The listing builds one solid part. Answer for the finished solid, in the listing's coordinates (mm). A direction names the side the tool comes from. Round coordinates to 2 decimals unless told otherwise and drop trailing zeros. Write each loop counter-clockwise with the first axis right and the second up, starting at its lowest first coordinate (ties: lowest second). Pieces come first, ordered by that corner, then holes. Notation, with made-up numbers: (3.25, -31) -> (37.25, -31) arc R26 ccw to (37.25, -12) -> close; hole circle Ø2 at (75, -20). An arc over 180 degrees is marked (long way). Write each question's results on one line, items separated by ' | '. Start each with the question number.
```python
from build123d import *

# Parameters (mm, degrees)
F1_DEPTH = 6
F2_R     = 6.5
F3_DEPTH = 6
F4_R     = 6.5
F5_DEPTH = 6


with BuildPart() as f1:
    # F0 (on Front) → F1 (new body)
    with BuildSketch(Plane.XZ):
        with BuildLine():
            Line((32, -12.5), (32, 12.5))
            Line((32, 12.5), (-32, 12.5))
            Line((-32, 12.5), (-32, 6.5))
            Line((-32, 6.5), (-12, 6.5))
            ThreePointArc((-12, 6.5), (-7.403806, 4.596194), (-5.5, 0))
            ThreePointArc((-5.5, 0), (-7.403806, -4.596194), (-12, -6.5))
            Line((-12, -6.5), (-32, -6.5))
            Line((-32, -6.5), (-32, -12.5))
            Line((-32, -12.5), (-12.5, -12.5))
            Line((-12.5, -12.5), (12.5, -12.5))
            Line((12.5, -12.5), (32, -12.5))
        make_face()
    extrude(amount=F1_DEPTH)

    # F2 (on face) → F3 (join)
    with BuildSketch(Plane.YZ.offset(32)):
        with BuildLine():
            Line((0, 12.5), (0, -12.5))
            Line((0, -12.5), (12, -12.5))
            ThreePointArc((12, -12.5), (24.5, 0), (12, 12.5))
            Line((12, 12.5), (0, 12.5))
        make_face()
        with Locations((12, 0)):
            Circle(F2_R, mode=Mode.SUBTRACT)
    extrude(amount=-F3_DEPTH)

    # F4 (on face) → F5 (join)
    with BuildSketch(Plane.XY.offset(12.5)):
        with BuildLine():
            Line((32, -18), (32, -6))
            Line((32, -6), (7, -6))
            Line((7, -6), (7, -18))
            ThreePointArc((7, -18), (19.5, -30.5), (32, -18))
        make_face()
        with Locations((19.5, -18)):
            Circle(F4_R, mode=Mode.SUBTRACT)
    extrude(amount=-F5_DEPTH)


solid = f1.part
```
Q1. Each of these flat-tipped pins is pushed along its axis until it touches: pin 1 (12.5 mm diameter, centred on x = 11, z = -6, fed in from +Y); pin 2 (8 mm diameter, centred on x = 12, y = -21, fed in from -Z); pin 3 (3 mm diameter, centred on x = -17, z = -6.5, fed in from -Y). Where does it stop, or does it pass through?
Q2. For faces 1 (the flat face through (-32, -3, -9)), 2 (the flat face through (25, -13, 6.5)), 3 (the flat face through (-22, -3, -6.5)), 4 (the flat face through (7, -12, 10)), 5 (the flat face through (26, 7, -5)), determine the directions among +Z, -Z, +X, -X, +Y, -Y from which every point of the face is accessible in a straight line to the end or side of a thin tool.
Q3. The part is cut by section D-D, the plane z = 9.75. Write down the section's boundary in (x, y), then the cut area to 3 significant figures.
Q4. The part is cut by section A-A, the plane x = -19. Write down the section's boundary in (y, z).
Q5. The part is cut by section B-B, the plane z = 3.75. Write down the section's boundary in (x, y), then the cut area to 3 significant figures.
Q6. The part is cut by section C-C, the plane y = -2.5. Write down the section's boundary in (x, z).
Q7. Determine the mould class of faces 6 (the flat face through (7, -6, 0)), 7 (the cylindrical face through (29.04, 18.2, 1.95)), 8 (the cylindrical face through (29.042, 24.497, -0.275)) for opening direction Z: pulls with the +Z half, pulls with the -Z half, needs draft (parallel to the pull), parting line crosses it, or undercut.
Q8. Find the intervals of material crossed by line 1 (Y direction, x = 19.5, z = 10.65); line 2 (Z direction, x = 27, y = 12); line 3 (Z direction, x = 10.5, y = -18), in increasing order.
Answers follow:
1) pin 1: y = 0 | pin 2: z = 6.5 | pin 3: y = -6
2) face 1: +Z, -Z, -X, +Y, -Y | face 2: -Z, +X, -X, -Y | face 3: -X, +Y, -Y | face 4: +Z, -Z, -X, -Y | face 5: +Z, -Z, -X, +Y
3) outline: (-32, -6) -> (7, -6) -> (7, -18) arc R12.5 ccw to (32, -18) -> (32, 19.82) -> (26, 19.82) -> (26, 0) -> (-32, 0) -> close; hole circle Ø13 at (19.5, -18) | area: 916 mm^2
4) outline: (-6, -12.5) -> (0, -12.5) -> (0, -6.5) -> (-6, -6.5) -> close; (-6, 6.5) -> (0, 6.5) -> (0, 12.5) -> (-6, 12.5) -> close
5) outline: (-6.69, -6) -> (32, -6) -> (32, 6.69) -> (26, 6.69) -> (26, 0) -> (-6.69, 0) -> close; (26, 17.31) -> (32, 17.31) -> (32, 23.92) -> (26, 23.92) -> close | area: 312 mm^2
6) outline: (-32, -12.5) -> (32, -12.5) -> (32, 12.5) -> (-32, 12.5) -> (-32, 6.5) -> (-12, 6.5) arc R6.5 cw to (-12, -6.5) -> (-32, -6.5) -> close
7) face 6: needs draft | face 7: undercut | face 8: parting line crosses it
8) line 1: -30.5 to -24.5, -11.5 to 0 | line 2: -12.5 to -6.5, 6.5 to 12.5 | line 3: 6.5 to 12.5
